```python
from build123d import *

# Parameters (mm, degrees)
F0_W     = 152.4
F0_H     = 152.4
F1_DEPTH = 25.4
F2_R     = 72.070602
F3_DEPTH = 25.4
F4_W     = 152.4
F4_H     = 152.73941
F5_DEPTH = 25.4


with BuildPart() as f1:
    # F0 (on Front) → F1 (new body)
    with BuildSketch(Plane.XZ):
        with Locations((-0.407152, -9.77602)):
            Rectangle(F0_W, F0_H)
    extrude(amount=F1_DEPTH)

    # F2 (on face) → F3 (join)
    with BuildSketch(Plane(origin=(0, 0, 0), x_dir=(-1, 0, 0), z_dir=(0, 1, 0))):
        Circle(F2_R)
    extrude(amount=F3_DEPTH)

    # F4 (on face) → F5 (join)
    with BuildSketch(Plane(origin=(0, 25.4, 0), x_dir=(-1, 0, 0), z_dir=(0, 1, 0))):
        with Locations((1.527745, -9.776019)):
            Rectangle(F4_W, F4_H)
    extrude(amount=F5_DEPTH)


solid = f1.part
```
Here's how the part is built. I have some questions about the finished solid (model axes, mm). A direction names the side the tool comes from. Coordinates: 2 decimals unless noted, no trailing zeros. Loops run counter-clockwise (first coordinate to the right, second up) from the corner with the lowest first, then second, coordinate; pieces in that order, holes last. Notation, with made-up numbers: (4, 18) - (23, 18) arc R19 ccw to (23, 35) - close; hole circle Ø3 at (1.25, 47.5). An arc over 180 degrees is marked (long way). Return JSON: item names as keys, results as strings. Group by question number.
Item 1: We'd pull the mould along Y, two halves only. Please class faces 1 (the face through (9.382, 12.522, 71.457)), 2 (the face through (0, 25.4, 69)), 3 (the face through (0, 38, 66.594)): +Y half, -Y half, draft (parallel to the pull), parting line (faces both ways), or undercut.
Item 2: If we section it at A-A on x = 0: Write out the boundary of the cut face in (y, z).
Item 3: Will these pins go through, and if not, where does the flat tip stop? P1, Ø8, axis at x = -60.5, y = 22.5, coming from the +Z side; P2, Ø10, axis at x = -2.5, y = 1.5, coming from the +Z side; P3, Ø12.5, axis at x = -37, y = -9, coming from the +Z side.
Item 4: If we section it at C-C on y = 4.5: Write out the boundary of the cut face in (x, z).
Item 5: On a 3-axis mill with a long thin cutter (end or side, diameter ignored), from which of +Z, -Z, +X, -X, +Y, -Y can I reach the whole of each face in a straight line? I mean faces 4 (the face through (-76.607, -13, -11)), 5 (the face through (-1, -13, 66.424)), 6 (the face through (74.672, 38, -11)), 7 (the face through (-7, 25.4, -77)). Say none if no direction works.
Item 6: I need wall thicknesses on line 1 (Y direction, x = -57.5, z = -69.5); line 2 (Z direction, x = 39.5, y = 30.5); line 3 (X direction, y = -21.5, z = 0.5). Which ranges of each line are inside material? Lowest first, please. Write a range as from..to.
Item 7: If we section it at B-B on z = 0: Write out the boundary of the cut face in (x, y).
Item 8: If we section it at D-D on y = 38.5: Write out the boundary of the cut face in (x, z).
Calculated:
{
 "1": {"face 1": "undercut", "face 2": "+Y half", "face 3": "draft"},
 "2": {"outline": "(-25.4, -85.98) - (0, -85.98) - (0, -72.07) - (25.4, -72.07) - (25.4, -86.15) - (50.8, -86.15) - (50.8, 66.59) - (25.4, 66.59) - (25.4, 72.07) - (0, 72.07) - (0, 66.42) - (-25.4, 66.42) - close"},
 "3": {"P1": "stops at z = 66.59", "P2": "stops at z = 72.07", "P3": "stops at z = 66.42"},
 "4": {"outline": "circle Ø144.14 at (0, 0)"},
 "5": {"face 4": "+Z, -Z, -X, -Y", "face 5": "+Z, +X, -X, -Y", "face 6": "+Z, -Z, +X, +Y", "face 7": "none"},
 "6": {"line 1": "y = -25.4..0, 25.4..50.8", "line 2": "z = -86.15..66.59", "line 3": "x = -76.61..75.79"},
 "7": {"outline": "(-77.73, 25.4) - (-72.07, 25.4) - (-72.07, 0) - (-76.61, 0) - (-76.61, -25.4) - (75.79, -25.4) - (75.79, 0) - (72.07, 0) - (72.07, 25.4) - (74.67, 25.4) - (74.67, 50.8) - (-77.73, 50.8) - close"},
 "8": {"outline": "(-77.73, -86.15) - (74.67, -86.15) - (74.67, 66.59) - (-77.73, 66.59) - close"}
}
